from build123d import *

# Parameters (mm, degrees)
SKETCH1_W           = 43
SKETCH1_H           = 49
SKETCH1_R           = 2.875
BOSS_EXTRUDE1_DEPTH = 6.75
SKETCH2_W           = 49
SKETCH2_H           = 5
BOSS_EXTRUDE2_DEPTH = 5
SKETCH3_W           = 49
SKETCH3_H           = 5
BOSS_EXTRUDE3_DEPTH = 5
SKETCH4_W           = 7
SKETCH4_H           = 5
BOSS_EXTRUDE4_DEPTH = 5
CHAMFER1_SIZE       = 2.5
FILLET1_R           = 0.5
SKETCH6_W           = 53
SKETCH6_H           = 3
BOSS_EXTRUDE6_DEPTH = 7
SKETCH7_R           = 1.9
CUT_EXTRUDE1_DEPTH  = 3
SKETCH9_W           = 34
SKETCH9_H           = 5
CUT_EXTRUDE2_DEPTH  = 5
SKETCH10_W          = 34
SKETCH10_H          = 5
CUT_EXTRUDE3_DEPTH  = 5
CHAMFER2_SIZE       = 3
FILLET2_R           = 3


with BuildPart() as part:
    # Sketch1 → Boss-Extrude1 (new body)
    with BuildSketch(Plane(origin=(0, 0, 0), x_dir=(1, 0, 0), z_dir=(0, 1, 0))):
        with Locations((21.5, -24.5)):
            Rectangle(SKETCH1_W, SKETCH1_H)
        with Locations((21.5, -20)):
            Circle(SKETCH1_R, mode=Mode.SUBTRACT)
    extrude(amount=BOSS_EXTRUDE1_DEPTH)

    # Sketch2 → Boss-Extrude2 (add)
    with BuildSketch(Plane.ZY):
        with Locations((24.5, 2.5)):
            Rectangle(SKETCH2_W, SKETCH2_H)
    extrude(amount=BOSS_EXTRUDE2_DEPTH)

    # Sketch3 → Boss-Extrude3 (add)
    with BuildSketch(Plane(origin=(43, 0, 0), x_dir=(0, 0, -1), z_dir=(1, 0, 0))):
        with Locations((-24.5, 2.5)):
            Rectangle(SKETCH3_W, SKETCH3_H)
    extrude(amount=BOSS_EXTRUDE3_DEPTH)

    # Sketch4 → Boss-Extrude4 (add)
    with BuildSketch(Plane(origin=(0, 0, 0), x_dir=(-1, 0, 0), z_dir=(0, 0, -1))):
        with Locations((-44.5, 2.5)):
            Rectangle(SKETCH4_W, SKETCH4_H)
        with Locations((1.5, 2.5)):
            Rectangle(SKETCH4_W, SKETCH4_H)
    extrude(amount=BOSS_EXTRUDE4_DEPTH)

    # Chamfer1
    chamfer1_edges = [part.edges().sort_by_distance(p)[0] for p in [
        (44.5, 0, -5),
        (-1.5, 0, -5),
    ]]
    chamfer(chamfer1_edges, length=CHAMFER1_SIZE)

    # Fillet1
    fillet1_edges = [part.edges().sort_by_distance(p)[0] for p in [
        (44.5, 5, -5),
        (-1.5, 5, -5),
    ]]
    fillet(fillet1_edges, radius=FILLET1_R)

    # Sketch6 → Boss-Extrude6 (add)
    with BuildSketch(Plane.XY.offset(49)):
        with Locations((21.5, 1.5)):
            Rectangle(SKETCH6_W, SKETCH6_H)
    extrude(amount=BOSS_EXTRUDE6_DEPTH)

    # Sketch7 → Cut-Extrude1 (cut)
    with BuildSketch(Plane(origin=(0, 3, 0), x_dir=(1, 0, 0), z_dir=(0, 1, 0))):
        with Locations((0, -52.5)):
            Circle(SKETCH7_R)
        with Locations((43, -52.5)):
            Circle(SKETCH7_R)
    extrude(amount=-CUT_EXTRUDE1_DEPTH, mode=Mode.SUBTRACT)

    # Sketch9 → Cut-Extrude2 (cut)
    with BuildSketch(Plane.ZY.offset(5)):
        with Locations((22, 2.5)):
            Rectangle(SKETCH9_W, SKETCH9_H)
    extrude(amount=-CUT_EXTRUDE2_DEPTH, mode=Mode.SUBTRACT)

    # Sketch10 → Cut-Extrude3 (cut)
    with BuildSketch(Plane(origin=(48, 0, 0), x_dir=(0, 0, -1), z_dir=(1, 0, 0))):
        with Locations((-22, 2.5)):
            Rectangle(SKETCH10_W, SKETCH10_H)
    extrude(amount=-CUT_EXTRUDE3_DEPTH, mode=Mode.SUBTRACT)

    # Chamfer2
    chamfer2_edges = [part.edges().sort_by_distance(p)[0] for p in [
        (-2.5, 0, 5),
        (-2.5, 0, 39),
        (45.5, 0, 39),
        (45.5, 0, 5),
    ]]
    chamfer(chamfer2_edges, length=CHAMFER2_SIZE)

    # Fillet2
    fillet2_edges = [part.edges().sort_by_distance(p)[0] for p in [
        (-5, 1.5, 56),
        (48, 1.5, 56),
    ]]
    fillet(fillet2_edges, radius=FILLET2_R)


solid = part.part
Input: part model. Units: mm. Frame: model coordinates. A direction names the side the tool comes from. Give positions to 0.01 mm unless a question says otherwise; leave off trailing zeros. Order: outer loops, then holes, each group sorted by start corner. A loop starts at its lowest first (then second) coordinate and runs counter-clockwise, first axis right, second up.
Q1. Ray query, probe 1 along X at (y, z) = (1.4, 52.5); probe 2 along X at (y, z) = (3.75, 20) (3 decimals); probe 3 along Z at (x, y) = (21.5, 4.75) (3 decimals). Return the intervals inside material, ascending.
Checked values:
probe 1: x = -5 to -1.9, 1.9 to 41.1, 44.9 to 48
probe 2: x = 0 to 18.625, 24.375 to 43
probe 3: z = 0 to 17.125, 22.875 to 49
Q2. Section B-B on y = 1.25. Output: boundary loops of the cut face in (x, z) (3 decimals), and give its area (3 significant figures).
Checked values:
outline: (-5, -3.75) - (2, -3.75) - (2, 0) - (41, 0) - (41, -3.75) - (48, -3.75) - (48, 3.25) - (43, 3.25) - (43, 40.75) - (48, 40.75) - (48, 53) arc R3 ccw to (45, 56) - (-2, 56) arc R3 ccw to (-5, 53) - (-5, 40.75) - (0, 40.75) - (0, 3.25) - (-5, 3.25) - close; hole circle Ø3.8 at (0, 52.5); hole circle Ø5.75 at (21.5, 20); hole circle Ø3.8 at (43, 52.5)
area: 2,590 mm2
Q3. Contact query for flat-ended pins moving along their axis: pin 1 Ø1.6 at (x, y) = (45.5, 4) entering from +Z; pin 2 Ø4 at (x, z) = (-3, 42) entering from +Y; pin 3 Ø4.5 at (x, z) = (0, 52.5) entering from +Y. Output: stop coordinate, or through.
Checked values:
pin 1: stops at z = 49
pin 2: stops at y = 5
pin 3: stops at y = 3
Q4. Set-up query: faces 1 (the flat face through (21, 3, 52)), 2 (the flat face through (46, 5, 44)), 3 (the flat face through (-3, 4, 39)). Return all of +Z, -Z, +X, -X, +Y, -Y with unobstructed straight access to the full face (end or side cutting, diameter ignored); none if empty.
Checked values:
face 1: +Z, +X, -X, +Y
face 2: +Z, -Z, +X, +Y
face 3: -X, +Y, -Y
Q5. Section D-D on z = 3. Output: boundary loops of the cut face in (x, y), and give its area (3 significant figures).
Checked values:
outline: (-5, 1) - (0, 1) - (0, 0) - (43, 0) - (43, 1) - (48, 1) - (48, 5) - (43, 5) - (43, 6.75) - (0, 6.75) - (0, 5) - (-5, 5) - close
area: 330 mm2
Q6. Draft query along X for faces 4 (the flat face through (-5, 2, 0)), 5 (the flat face through (-3, 2, 4)), 6 (the flat face through (2, 2, -2)). Return one class per face: +X half, -X half, draft (parallel to the pull), parting line (faces both ways), or undercut.
Checked values:
face 4: -X half
face 5: draft
face 6: undercut
Q7. Section A-A on x = 21.5. Output: boundary loops of the cut face in (y, z) (3 decimals).
Checked values:
outline: (0, 0) - (6.75, 0) - (6.75, 17.125) - (0, 17.125) - close; (0, 22.875) - (6.75, 22.875) - (6.75, 49) - (3, 49) - (3, 56) - (0, 56) - close
Q8. Section C-C on z = 20. Output: boundary loops of the cut face in (x, y) (3 decimals), and give its area (3 significant figures).
Checked values:
outline: (0, 0) - (18.625, 0) - (18.625, 6.75) - (0, 6.75) - close; (24.375, 0) - (43, 0) - (43, 6.75) - (24.375, 6.75) - close
area: 251 mm2
